Verification items for the finished model (mm, model axes). Face numbers are marked on the shaded views. A direction names the side the tool comes from. Round coordinates to 2 decimals unless told otherwise and drop trailing zeros. Order: outer loops, then holes, each group sorted by start corner. A loop starts at its lowest first (then second) coordinate and runs counter-clockwise, first axis right, second up. Notation, with made-up numbers: (76.5, 41.25) -> (133.5, 41.25) arc R24 ccw to (133.5, 59.25) -> close; hole circle Ø5 at (13.25, 38). An arc over 180 degrees is marked (long way). Put each result on its own line as item: value.
from build123d import *

# Parameters (mm, degrees)
F0_R      = 5.5
F1_DEPTH  = 13
F2_W      = 19
F2_H      = 32
F3_DEPTH  = 64
F4_R      = 6.5
F5_DEPTH  = 19
F6_W      = 17
F6_H      = 32
F7_DEPTH  = 30
F10_W     = 35
F10_H     = 17
F11_DEPTH = 32


with BuildPart() as f1:
    # F0 (on Top) → F1 (new body)
    with BuildSketch(Plane.XY):
        Polygon((0, 32), (0, 0), (15, 0), (25, 10), (25, 32), align=None)
        with Locations((13, 16)):
            Circle(F0_R, mode=Mode.SUBTRACT)
    extrude(amount=F1_DEPTH)

    # F2 (on Top) → F3 (join)
    with BuildSketch(Plane.XY):
        with Locations((-9.5, 16)):
            Rectangle(F2_W, F2_H)
    extrude(amount=F3_DEPTH)

    # F4 (on face) → F5 (cut, through all)
    with BuildSketch(Plane.YZ):
        with Locations((16, 46)):
            Circle(F4_R)
    extrude(amount=-F5_DEPTH, mode=Mode.SUBTRACT)

    # F6 (on Top) → F7 (join)
    with BuildSketch(Plane.XY):
        with Locations((-27.5, 16)):
            Rectangle(F6_W, F6_H)
    extrude(amount=F7_DEPTH)

    # F9: F1 across plane


with BuildPart() as f1_1:
    add(f1.part)
    add(f1.part.mirror(Plane(origin=(-36, 16, 15), x_dir=(0, -1, 0), z_dir=(-1, 0, 0))))

    # F10 (on face) → F11 (cut, through all)
    with BuildSketch(Plane.XZ):
        with Locations((-31.5, 8.5)):
            Rectangle(F10_W, F10_H)
    extrude(amount=-F11_DEPTH, mode=Mode.SUBTRACT)


solid = f1_1.part
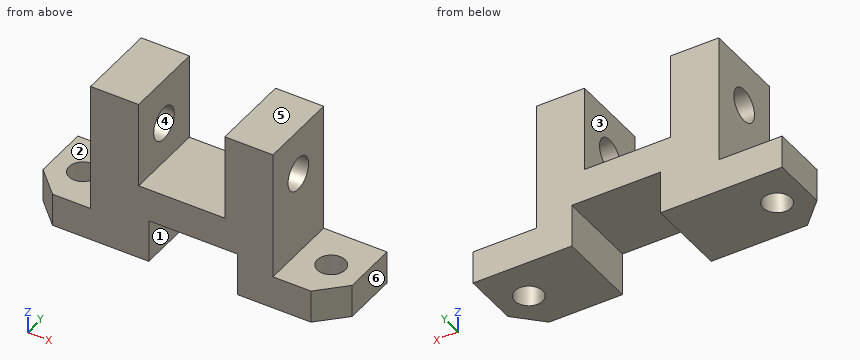
Item 1: Section check C-C on x = 13. Record the boundary of the cut face in (y, z), then the cut area to 3 significant figures.
Check sheet entries:
outline: (0, 0) -> (10.5, 0) -> (10.5, 13) -> (0, 13) -> close; (21.5, 0) -> (32, 0) -> (32, 13) -> (21.5, 13) -> close
area: 273 mm^2
Item 2: Section check D-D on z = 46. Record the boundary of the cut face in (x, y), then the cut area to 3 significant figures.
Check sheet entries:
outline: (-72, 0) -> (-53, 0) -> (-53, 9.5) -> (-72, 9.5) -> close; (-72, 22.5) -> (-53, 22.5) -> (-53, 32) -> (-72, 32) -> close; (-19, 0) -> (0, 0) -> (0, 9.5) -> (-19, 9.5) -> close; (-19, 22.5) -> (0, 22.5) -> (0, 32) -> (-19, 32) -> close
area: 722 mm^2
Item 3: Section check A-A on y = 16. State how many separate pieces and enclosed holes the cut face has, then the cut area to 3 significant figures.
Check sheet entries:
separate pieces: 5
enclosed holes: 0
area: 2,730 mm^2
Item 4: Material ranges on L1, parallel to Z at x = -64.75, y = 16; L2, parallel to Y at x = -85, z = 9; L3, parallel to X at y = 22.5, z = 58, recorded low to high. Write a range as [from, to].
Check sheet entries:
L1: z = [0, 39.5], [52.5, 64]
L2: y = [0, 10.5], [21.5, 32]
L3: x = [-72, -53], [-19, 0]
Item 5: Release check for a two-part mould opening along Z. For the marked faces 4, 5 and 6 record: +Z half, -Z half, draft (parallel to the pull), parting line (faces both ways), or undercut.
Check sheet entries:
face 4: undercut
face 5: +Z half
face 6: draft
Item 6: Tool access check on the marked faces 1, 2 and 3. Record the directions out of +Z, -Z, +X, -X, +Y, -Y that give a thin tool (end or side, any length) a straight path to the whole face; none if there is none.
Check sheet entries:
face 1: -Z, +Y, -Y
face 2: +Z, -X, +Y, -Y
face 3: +Z, +Y, -Y
Item 7: Section check B-B on z = 6. Record the boundary of the cut face in (x, y).
Check sheet entries:
outline: (-97, 10) -> (-87, 0) -> (-49, 0) -> (-49, 32) -> (-97, 32) -> close; (-14, 0) -> (15, 0) -> (25, 10) -> (25, 32) -> (-14, 32) -> close; hole circle Ø11 at (-85, 16); hole circle Ø11 at (13, 16)
Item 8: Gauge pin test, flat ends, axial feed: pin 1 Ø17 at (y, z) = (16, 46) entering from +X; pin 2 Ø12 at (x, y) = (-29, 21) entering from +Z; pin 3 Ø9.5 at (y, z) = (14, 27.5) entering from -X; pin 4 Ø12 at (x, y) = (-68.5, 14.5) entering from -Z. Record the tip position at first contact, or that the pin passes through.
Check sheet entries:
pin 1: stops at x = 0
pin 2: stops at z = 30
pin 3: stops at x = -72
pin 4: stops at z = 0
